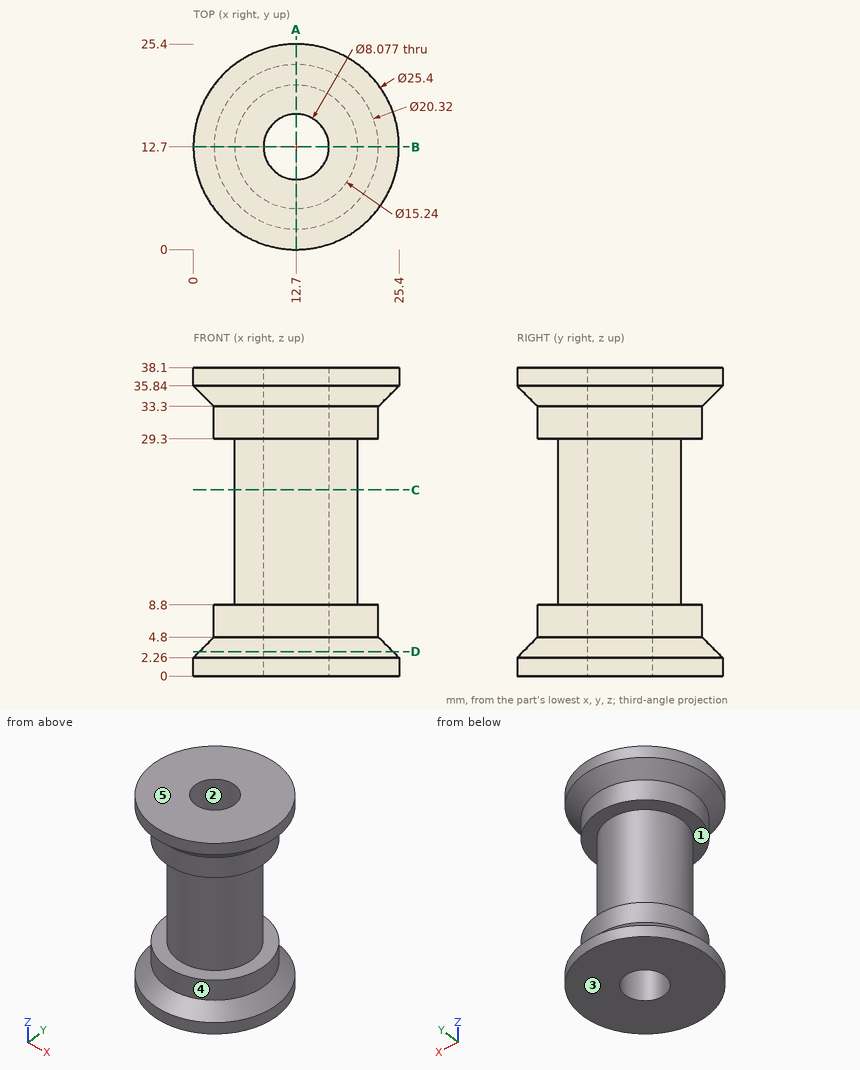
The figure shows three views and two pictorial views of one solid part (mm, origin at its lowest corner). Answer the questions. A direction names the side the tool comes from. Coordinates: 2 decimals unless noted, no trailing zeros. Order: outer loops, then holes, each group sorted by start corner. A loop starts at its lowest first (then second) coordinate and runs counter-clockwise, first axis right, second up. Notation, with made-up numbers: (5, -39) - (23, -39) arc R9 ccw to (23, -34) - close; hole circle Ø10 at (-22, -23.5). An arc over 180 degrees is marked (long way). Answer as a JSON object with one key per item and string values.
1. Find section C-C on z = 23. Determine the outline of the cut face in (x, y).
Output values:
{"outline": "circle Ø15.24 at (12.7, 12.7); hole circle Ø8.08 at (12.7, 12.7)"}
2. Find section D-D on z = 3. Determine the outline of the cut face in (x, y), plus the area to 3 significant figures.
Output values:
{"outline": "circle Ø23.92 at (12.7, 12.7); hole circle Ø8.08 at (12.7, 12.7)", "area": "398 mm²"}
3. Each of these flat-tipped pins is pushed along its axis until it touches: P1, Ø1, axis at x = 21, z = 9.5, coming from the -Y side; P2, Ø1.5, axis at y = 5.5, z = 33.5, coming from the +X side; P3, Ø8, axis at y = 7, z = 19.5, coming from the +X side; P4, Ø4, axis at y = 19, z = 21, coming from the -X side. Where does it stop, or does it pass through?
Output values:
{"P1": "passes through", "P2": "stops at x = 21.34", "P3": "stops at x = 20.13", "P4": "stops at x = 6.41"}
4. A tool of negligible diameter and unlimited length cuts with its end or side. For the marked faces 4 and 5, from which of +Z, -Z, +X, -X, +Y, -Y can it reach the whole face along a straight path? Write none if from no direction.
Output values:
{"face 4": "none", "face 5": "+Z, +X, -X, +Y, -Y"}
5. Find section A-A on x = 12.7. Determine the outline of the cut face in (y, z).
Output values:
{"outline": "(0, 0) - (8.66, 0) - (8.66, 38.1) - (0, 38.1) - (0, 35.84) - (2.54, 33.3) - (2.54, 29.3) - (5.08, 29.3) - (5.08, 8.8) - (2.54, 8.8) - (2.54, 4.8) - (0, 2.26) - close; (16.74, 0) - (25.4, 0) - (25.4, 2.26) - (22.86, 4.8) - (22.86, 8.8) - (20.32, 8.8) - (20.32, 29.3) - (22.86, 29.3) - (22.86, 33.3) - (25.4, 35.84) - (25.4, 38.1) - (16.74, 38.1) - close"}
6. Consider line 1 (Z direction, x = 4, y = 15.5); line 2 (Y direction, x = 12.7, z = 16); line 3 (Y direction, x = 12.7, z = 30). Determine where each line is inside the solid, lowest interval first.
Output values:
{"line 1": "z = 0 to 8.8, 29.3 to 38.1", "line 2": "y = 5.08 to 8.66, 16.74 to 20.32", "line 3": "y = 2.54 to 8.66, 16.74 to 22.86"}
7. The mould has two halves that part along Z. Classify the marked faces 1, 2 and 3: +Z half, -Z half, draft (parallel to the pull), parting line (faces both ways), or undercut.
Output values:
{"face 1": "undercut", "face 2": "draft", "face 3": "-Z half"}
